```python
from build123d import *

# Parameters (mm, degrees)
CROQUIS1_W              = 111
CROQUIS1_H              = 64
CROQUIS1_R              = 1.375
SALIENTE_EXTRUIR1_DEPTH = 5
CROQUIS2_W              = 5
CROQUIS2_H              = 21.333333334
SALIENTE_EXTRUIR2_DEPTH = 5
CROQUIS3_W              = 5
CROQUIS3_H              = 21.333333334
SALIENTE_EXTRUIR3_DEPTH = 5


with BuildPart() as part:
    # Croquis1 → Saliente-Extruir1 (new body)
    with BuildSketch(Plane.XY):
        with Locations((12.5, -8)):
            Rectangle(CROQUIS1_W, CROQUIS1_H)
        with Locations((42.920083817, -32.303397977)):
            Circle(CROQUIS1_R, mode=Mode.SUBTRACT)
        with Locations((42.920083817, 16.696602023)):
            Circle(CROQUIS1_R, mode=Mode.SUBTRACT)
        with Locations((-15.079916183, -32.303397977)):
            Circle(CROQUIS1_R, mode=Mode.SUBTRACT)
        with Locations((-15.079916183, 16.696602023)):
            Circle(CROQUIS1_R, mode=Mode.SUBTRACT)
        with BuildLine():
            Line((60.939336221, 9.212655439), (-11.729916183, 9.212655439))
            ThreePointArc((-11.729916183, 9.212655439), (-13.325171123, 10.807910378), (-11.729916183, 12.403165318))
            Line((-11.729916183, 12.403165318), (60.939336221, 12.403165318))
            ThreePointArc((60.939336221, 12.403165318), (62.53459116, 10.807910378), (60.939336221, 9.212655439))
        make_face(mode=Mode.SUBTRACT)
        with BuildLine():
            Line((60.939336221, 3.212655439), (-11.729916183, 3.212655439))
            ThreePointArc((-11.729916183, 3.212655439), (-13.325171123, 4.807910378), (-11.729916183, 6.403165318))
            Line((-11.729916183, 6.403165318), (60.939336221, 6.403165318))
            ThreePointArc((60.939336221, 6.403165318), (62.53459116, 4.807910378), (60.939336221, 3.212655439))
        make_face(mode=Mode.SUBTRACT)
        with BuildLine():
            Line((60.939336221, -2.787344561), (-11.729916183, -2.787344561))
            ThreePointArc((-11.729916183, -2.787344561), (-13.325171123, -1.192089622), (-11.729916183, 0.403165318))
            Line((-11.729916183, 0.403165318), (60.939336221, 0.403165318))
            ThreePointArc((60.939336221, 0.403165318), (62.53459116, -1.192089622), (60.939336221, -2.787344561))
        make_face(mode=Mode.SUBTRACT)
        with BuildLine():
            Line((60.939336221, -8.787344561), (-11.729916183, -8.787344561))
            ThreePointArc((-11.729916183, -8.787344561), (-13.325171123, -7.192089622), (-11.729916183, -5.596834682))
            Line((-11.729916183, -5.596834682), (60.939336221, -5.596834682))
            ThreePointArc((60.939336221, -5.596834682), (62.53459116, -7.192089622), (60.939336221, -8.787344561))
        make_face(mode=Mode.SUBTRACT)
        with BuildLine():
            Line((60.939336221, -14.787344561), (-11.729916183, -14.787344561))
            ThreePointArc((-11.729916183, -14.787344561), (-13.325171123, -13.192089622), (-11.729916183, -11.596834682))
            Line((-11.729916183, -11.596834682), (60.939336221, -11.596834682))
            ThreePointArc((60.939336221, -11.596834682), (62.53459116, -13.192089622), (60.939336221, -14.787344561))
        make_face(mode=Mode.SUBTRACT)
        with BuildLine():
            Line((60.939336221, -20.787344561), (-11.729916183, -20.787344561))
            ThreePointArc((-11.729916183, -20.787344561), (-13.325171123, -19.192089622), (-11.729916183, -17.596834682))
            Line((-11.729916183, -17.596834682), (60.939336221, -17.596834682))
            ThreePointArc((60.939336221, -17.596834682), (62.53459116, -19.192089622), (60.939336221, -20.787344561))
        make_face(mode=Mode.SUBTRACT)
        with BuildLine():
            Line((60.939336221, -26.787344561), (-11.729916183, -26.787344561))
            ThreePointArc((-11.729916183, -26.787344561), (-13.325171123, -25.192089622), (-11.729916183, -23.596834682))
            Line((-11.729916183, -23.596834682), (60.939336221, -23.596834682))
            ThreePointArc((60.939336221, -23.596834682), (62.53459116, -25.192089622), (60.939336221, -26.787344561))
        make_face(mode=Mode.SUBTRACT)
    extrude(amount=SALIENTE_EXTRUIR1_DEPTH)

    # Croquis2 → Saliente-Extruir2 (add)
    with BuildSketch(Plane(origin=(68, 0, 0), x_dir=(0, 0, -1), z_dir=(1, 0, 0))):
        with Locations((-2.5, -8)):
            Rectangle(CROQUIS2_W, CROQUIS2_H)
    extrude(amount=SALIENTE_EXTRUIR2_DEPTH)

    # Croquis3 → Saliente-Extruir3 (add)
    with BuildSketch(Plane.ZY.offset(43)):
        with Locations((2.5, -8)):
            Rectangle(CROQUIS3_W, CROQUIS3_H)
    extrude(amount=SALIENTE_EXTRUIR3_DEPTH)


solid = part.part
```
Can you work these out from the model? Positions are in its coordinate system, mm. A direction names the side the tool comes from. Coordinates: 2 decimals unless noted, no trailing zeros. Loops run counter-clockwise (first coordinate to the right, second up) from the corner with the lowest first, then second, coordinate; pieces in that order, holes last. Notation, with made-up numbers: (9.5, 46) -> (48.5, 46) arc R31 ccw to (48.5, 77) -> close; hole circle Ø9 at (-35.5, 48.5). An arc over 180 degrees is marked (long way). Put each result on its own line as item: value. Start each with the question number.
Q1. I'm going to push flat-ended pins straight in: P1, Ø1.5, axis at x = -45, z = 3, coming from the +Y side; P2, Ø1.5, axis at x = 71, z = 2.5, coming from the -Y side; P3, Ø3, axis at y = -20.5, z = 3.5, coming from the +X side. Where does each tip first touch, or does it pass through?
Q2. I want a section at B-B (y = -7.5). Write out the boundary of the cut face in (x, z), plus the area to 3 significant figures.
Q3. If I drill on line 1 (X direction, y = -29.5, z = 2.1); line 2 (Y direction, x = -16, z = 3.25); line 3 (X direction, y = -20, z = 1.1), over which ranges is the centre line in solid material (lowest first)? Write a range as [from, to].
Q4. For faces 5 (the face through (-48, -8, 2)), 6 (the face through (25, -2.787, 2)), 7 (the face through (70, -18.667, 3)), 8 (the face through (70, 2.667, 3)), which set-ups out of +Z, -Z, +X, -X, +Y, -Y let a thin tool reach every point of the face, with its end or its side?
Q5. Thinking about a two-plate mould opening in Y: for faces 1 (the face through (-45, -18.667, 2)), 2 (the face through (68, -29, 2)), 3 (the face through (-45, 2.667, 2)), 4 (the face through (-15.378, 15.354, 2.465)), which applies, pulls with the +Y half, pulls with the -Y half, needs draft (parallel to the pull), parting line crosses it, or undercut?
Q6. I want a section at A-A (x = 14). Count the separate pieces of the cut face and the enclosed holes in it, plus the area to 3 significant figures.
Taken from the geometry:
1. P1: stops at y = 2.67
1. P2: stops at y = -18.67
1. P3: stops at x = 68
2. outline: (-48, 0) -> (-13.3, 0) -> (-13.3, 5) -> (-48, 5) -> close; (62.5, 0) -> (73, 0) -> (73, 5) -> (62.5, 5) -> close
2. area: 226 mm2
3. line 1: x = [-43, 68]
3. line 2: y = [-40, -33.33], [-31.28, 15.67], [17.72, 24]
3. line 3: x = [-43, -13.11], [62.31, 68]
4. face 5: +Z, -Z, -X, +Y, -Y
4. face 6: +Z, -Z
4. face 7: +Z, -Z, +X, -Y
4. face 8: +Z, -Z, +X, +Y
5. face 1: pulls with the -Y half
5. face 2: needs draft
5. face 3: pulls with the +Y half
5. face 4: undercut
6. separate pieces: 8
6. enclosed holes: 0
6. area: 208 mm2
